Can you work these out from the model? Positions are in its coordinate system, mm. Give positions to 0.01 mm unless a question says otherwise; leave off trailing zeros. Write each loop counter-clockwise with the first axis right and the second up, starting at its lowest first coordinate (ties: lowest second). Pieces come first, ordered by that corner, then holes.
Autodesk Inventor part; units mm, degrees
ref_plane "YZ Plane" through (0, 0, 0) normal (1, 0, 0) x (0, 1, 0)
ref_plane "XZ Plane" through (0, 0, 0) normal (0, 1, 0) x (-1, 0, 0)
ref_plane "XY Plane" through (0, 0, 0) normal (0, 0, 1) x (1, 0, 0)
sketch "スケッチ6" plane through (0, 0, 0) normal (0, 0, 1) x (1, 0, 0)
  line L0 (30, 10) -> (30, 100)
  line L1 (30, 100) -> (0, 100)
  line L2 (0, 100) -> (0, 0)
  line L3 (0, 100) -> (-10, 100)
  line L4 (-10, 100) -> (-10, 90)
  line L5 (-10, 90) -> (0, 90)
  line L6 (0, 90) -> (0, 100)
  line L7 (30, 100) -> (40, 100)
  line L8 (40, 100) -> (40, 90)
  line L9 (40, 90) -> (30, 90)
  line L10 (30, 90) -> (30, 100)
  line L11 (0, 50) -> (-10, 50)
  line L12 (-10, 50) -> (-10, 60)
  line L13 (-10, 60) -> (0, 60)
  line L14 (0, 60) -> (0, 50)
  line L15 (30, 50) -> (40, 50)
  line L16 (40, 50) -> (40, 60)
  line L17 (40, 60) -> (30, 60)
  line L18 (30, 60) -> (30, 50)
  line L19 (0, 20) -> (-10, 20)
  line L20 (-10, 20) -> (-10, 10)
  line L21 (-10, 10) -> (0, 10)
  line L22 (0, 10) -> (0, 20)
  line L23 (30, 20) -> (40, 20)
  line L24 (40, 20) -> (40, 10)
  line L25 (40, 10) -> (30, 10)
  line L26 (30, 10) -> (30, 20)
  line L27 (0, 100) -> (30, 100)
  line L28 (30, 100) -> (30, 10)
  line L29 (30, 10) -> (0, 10)
  line L30 (0, 10) -> (0, 100)
  line L31 (-10, 100) -> (40, 100)
  line L32 (40, 100) -> (40, 10)
  line L33 (40, 10) -> (-10, 10)
  line L34 (-10, 10) -> (-10, 100)
  point P0 (0, 90)
  point P1 (30, 55)
  point P2 (0, 10)
  point P3 (0, 10)
  point P4 (0, 60)
  dimension "d73" = 30
  dimension "d117" = 10
  dimension "d118" = 10
  dimension "d119" = 10
  dimension "d120" = 10
  dimension "d141" = 10
  dimension "d142" = 0
  dimension "d143" = 30
  dimension "d144" = 10
  dimension "d145" = 10
  dimension "d146" = 10
  dimension "d147" = 10
  dimension "d149" = 30
  dimension "d167" = 90
extrude "押し出し5" add sketch "スケッチ6" along normal blind 3
sketch "スケッチ7" plane through (0, 0, 3) normal (0, 0, 1) x (1, 0, 0)
  line L0 (30, 90) -> (30, 90)
  circle A0 centre (15, 85) radius 6
  line L1 (15, 85) -> (15, 104.27)
  line L2 (40, 100) -> (-10, 100)
  point P0 (0, 0)
  point P1 (30, 0)
  point P2 (15, 91)
  point P3 (9, 85)
  point P4 (15, 79)
  point P5 (21, 85)
  point P6 (30, 10)
  point P7 (15, 100)
  dimension "d79" = 12
  dimension "d82" = 360
  dimension "d156" = 0
hole "穴2" at (15, 85, 3) at (15, 91, 3) at (9, 85, 3) at (15, 79, 3) at (21, 85, 3) direction (0, 0, -1) diameter 1.5 end through all
sketch "スケッチ8" plane through (0, 0, 3) normal (0, 0, 1) x (1, 0, 0)
  line L0 (5, 69) -> (25, 69)
  line L1 (25, 69) -> (25, 15)
  line L2 (25, 15) -> (5, 15)
  line L3 (5, 15) -> (5, 69)
  line L4 (5, 62.45) -> (25, 62.45)
  line L5 (25, 62.45) -> (25, 21.55)
  line L6 (25, 21.55) -> (5, 21.55)
  line L7 (5, 21.55) -> (5, 62.45)
  circle A0 centre (10, 66.3) radius 1.95
  circle A1 centre (20, 66.3) radius 1.95
  circle A2 centre (10, 17.7) radius 1.95
  circle A3 centre (20, 17.7) radius 1.95
  line L8 (-10, 10) -> (40, 10)
  line L9 (-10, 100) -> (-10, 10)
  point P0 (0, 100)
  point P1 (15, 21.55)
  point P2 (25, 62.45)
  dimension "d91" = 20
  dimension "d93" = 54
  dimension "d96" = 10
  dimension "d98" = 48.6
  dimension "d99" = 2.7
  dimension "d100" = 5
  dimension "d101" = 40.9
  dimension "d102" = 6.55
  dimension "d105" = 3.9
  dimension "d106" = 3.9
  dimension "d107" = 3.9
  dimension "d151" = 3.9
  dimension "d152" = 10
  dimension "d153" = 5
  dimension "d154" = 2.7
  dimension "d168" = 5
  dimension "d169" = 15
extrude "押し出し6" cut sketch "スケッチ8" against normal blind 3 contours L4 L1 L6 L3 | A0 | A1 | A2 | A3
sketch "スケッチ9" plane through (0, 0, 3) normal (0, 0, 1) x (1, 0, 0)
  line L0 (-10, 100) -> (-10, 10)
  line L1 (40, 90) -> (40, 100)
  line L2 (40, 100) -> (-10, 100)
  line L3 (0, 60) -> (-10, 60)
  line L4 (40, 60) -> (30, 60)
  line L5 (40, 50) -> (40, 60)
  line L6 (-10, 60) -> (-10, 50)
  line L7 (-10, 20) -> (-10, 10)
  line L8 (0, 20) -> (-10, 20)
  line L9 (40, 20) -> (30, 20)
  line L10 (40, 10) -> (40, 20)
  point P0 (-5, 95)
  point P1 (35, 95)
  point P2 (-10, 90)
  point P3 (40, 95)
  point P4 (-5, 55)
  point P5 (35, 55)
  point P6 (35, 15)
  point P7 (-5, 15)
  dimension "d126" = 5
  dimension "d127" = 5
  dimension "d157" = 5
  dimension "d158" = 5
  dimension "d159" = 5
  dimension "d160" = 5
  dimension "d161" = 5
  dimension "d162" = 5
  dimension "d163" = 5
  dimension "d164" = 5
  dimension "d165" = 5
  dimension "d166" = 5
hole "穴3" at (-5, 95, 3) at (35, 95, 3) at (-5, 55, 3) at (35, 55, 3) at (35, 15, 3) at (-5, 15, 3) direction (0, 0, -1) diameter 3 end through all
equation "\"d120\" = d119"
equation "\"d141\" = d120"
equation "\"d144\" = d120"
equation "\"d145\" = d144"
equation "\"d147\" = d141"
equation "\"d149\" = d143"
equation "\"d151\" = d107"
properties part number "practice_parts01"
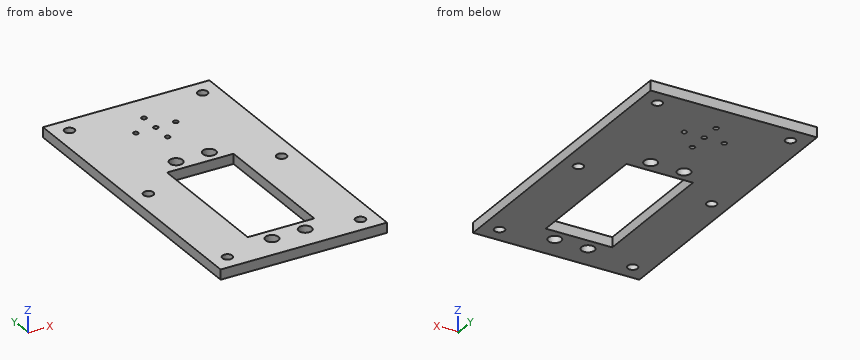
1) Suppose I cut it at B-B on z = 1.4. State how many separate pieces and enclosed holes the cut face has, plus the area to 3 significant figures.
Values follow:
separate pieces: 1
enclosed holes: 16
area: 3,580 mm2
2) Please list where these lines run through material, in increasing order: L1, parallel to Y at x = 20, z = 0.95; L2, parallel to Y at x = 35, z = 0.85; L3, parallel to X at y = 85, z = 2.3.
Values follow:
L1: y = 10 to 15.75, 19.65 to 21.55, 62.45 to 64.35, 68.25 to 100
L2: y = 10 to 13.5, 16.5 to 53.5, 56.5 to 93.5, 96.5 to 100
L3: x = -10 to 8.25, 9.75 to 14.25, 15.75 to 20.25, 21.75 to 40
3) Suppose I cut it at C-C on y = 17.7. Write out the boundary of the cut face in (x, z), plus the area to 3 significant figures.
Values follow:
outline: (-10, 0) - (8.05, 0) - (8.05, 3) - (-10, 3) - close; (11.95, 0) - (18.05, 0) - (18.05, 3) - (11.95, 3) - close; (21.95, 0) - (40, 0) - (40, 3) - (21.95, 3) - close
area: 127 mm2
4) Suppose I cut it at A-A on y = 31. Write out the boundary of the cut face in (x, z).
Values follow:
outline: (-10, 0) - (5, 0) - (5, 3) - (-10, 3) - close; (25, 0) - (40, 0) - (40, 3) - (25, 3) - close
